```python
from build123d import *

# Parameters (mm, degrees)
SKETCH8_W                    = 28.7
SKETCH8_H                    = 15
BASE_FLANGE1_DEPTH           = 3.175
EDGE_FLANGE1_STRIP_W         = 16.7
EDGE_FLANGE1_STRIP_H         = 3.175
EDGE_FLANGE1_STRIP_CUT_DEPTH = 15
EDGE_FLANGE1_DEPTH           = 15
EDGE_FLANGE2_STRIP_W         = 16.7
EDGE_FLANGE2_STRIP_H         = 3.175
EDGE_FLANGE2_STRIP_CUT_DEPTH = 15
EDGE_FLANGE2_DEPTH           = 15
SKETCH19_R                   = 1.5
CUT_EXTRUDE1_DEPTH           = 10
CUT_EXTRUDE2_DEPTH           = 64.825465137
CUT_EXTRUDE2_DEPTH_BACK      = 64.825465137
CUT_EXTRUDE3_DEPTH           = 64.825465137
CUT_EXTRUDE3_DEPTH_BACK      = 64.825465137
SKETCH21_R                   = 1.5
FILLET1_R                    = 3


# Sheet-metal steps are written as plain solids
with BuildPart() as part:
    # Sketch8 → Base-Flange1 (new body)
    with BuildSketch(Plane(origin=(0, 0, 0), x_dir=(1, 0, 0), z_dir=(0, 1, 0))):
        with Locations((0, 7.5)):
            Rectangle(SKETCH8_W, SKETCH8_H)
    extrude(amount=-BASE_FLANGE1_DEPTH)

    # Edge-Flange1 strip (across the edge) → Edge-Flange1 strip cut (cut)
    with BuildSketch(Plane(origin=(14.35, -3.175, -15), x_dir=(-1, 0, 0), z_dir=(0, 0, 1))):
        with Locations((-3.175, -1.5875)):
            Rectangle(EDGE_FLANGE1_STRIP_W, EDGE_FLANGE1_STRIP_H)
    extrude(amount=EDGE_FLANGE1_STRIP_CUT_DEPTH, mode=Mode.SUBTRACT)

    # Edge-Flange1 section (across the edge) → Edge-Flange1 (add)
    with BuildSketch(Plane(origin=(14.35, -3.175, -15), x_dir=(-1, 0, 0), z_dir=(0, 0, 1))):
        with BuildLine():
            Line((0, 2), (0, 51.825))
            Line((0, 51.825), (3.175, 51.825))
            Line((3.175, 51.825), (3.175, 2))
            ThreePointArc((3.175, 2), (3.760786438, 0.585786438), (5.175, 0))
            Line((5.175, 0), (5.175, -3.175))
            ThreePointArc((5.175, -3.175), (1.515722407, -1.659277593), (0, 2))
        make_face()
    extrude(amount=EDGE_FLANGE1_DEPTH)

    # Edge-Flange2 strip (across the edge) → Edge-Flange2 strip cut (cut)
    with BuildSketch(Plane(origin=(-14.35, -3.175, 0), x_dir=(1, 0, 0), z_dir=(0, 0, -1))):
        with Locations((-3.175, -1.5875)):
            Rectangle(EDGE_FLANGE2_STRIP_W, EDGE_FLANGE2_STRIP_H)
    extrude(amount=EDGE_FLANGE2_STRIP_CUT_DEPTH, mode=Mode.SUBTRACT)

    # Edge-Flange2 section (across the edge) → Edge-Flange2 (add)
    with BuildSketch(Plane(origin=(-14.35, -3.175, 0), x_dir=(1, 0, 0), z_dir=(0, 0, -1))):
        with BuildLine():
            Line((0, 2), (0, 51.825))
            Line((0, 51.825), (3.175, 51.825))
            Line((3.175, 51.825), (3.175, 2))
            ThreePointArc((3.175, 2), (3.760786438, 0.585786438), (5.175, 0))
            Line((5.175, 0), (5.175, -3.175))
            ThreePointArc((5.175, -3.175), (1.515722407, -1.659277593), (0, 2))
        make_face()
    extrude(amount=EDGE_FLANGE2_DEPTH)

    # Sketch19 → Cut-Extrude1 (cut)
    with BuildSketch(Plane(origin=(0, 0, 0), x_dir=(1, 0, 0), z_dir=(0, 1, 0))):
        with Locations(Location((0, 7.5, 0), (0, 0, 270))):
            Circle(SKETCH19_R)
    extrude(amount=-CUT_EXTRUDE1_DEPTH, mode=Mode.SUBTRACT)

    # Sketch20 → Cut-Extrude2 (cut, two sides: drawn at the far end of the back side and taken through both)
    with BuildSketch(Plane(origin=(14.35, 0, 0), x_dir=(0, 0, -1), z_dir=(1, 0, 0)).offset(-CUT_EXTRUDE2_DEPTH_BACK)):
        Polygon((11.5, -55), (15, -5.175), (15, -55), align=None)
        Polygon((3.5, -55), (0, -5.175), (0, -55), align=None)
    extrude(amount=CUT_EXTRUDE2_DEPTH + CUT_EXTRUDE2_DEPTH_BACK, mode=Mode.SUBTRACT)

    # Sketch21 → Cut-Extrude3 (cut, two sides: drawn at the far end of the back side and taken through both)
    with BuildSketch(Plane(origin=(14.35, 0, 0), x_dir=(0, 0, -1), z_dir=(1, 0, 0)).offset(-CUT_EXTRUDE3_DEPTH_BACK)):
        with Locations(Location((7.5, -50.5, 0), (0, 0, 90))):
            Circle(SKETCH21_R)
    extrude(amount=CUT_EXTRUDE3_DEPTH + CUT_EXTRUDE3_DEPTH_BACK, mode=Mode.SUBTRACT)

    # Fillet1
    fillet1_edges = [part.edges().sort_by_distance(p)[0] for p in [
        (12.7625, -55, -3.5),
        (12.7625, -55, -11.5),
        (-12.7625, -55, -3.5),
        (-12.7625, -55, -11.5),
    ]]
    fillet(fillet1_edges, radius=FILLET1_R)


solid = part.part
```
The listing builds one solid part. Answer for the finished solid, in the listing's coordinates (mm). A direction names the side the tool comes from. Coordinates: 2 decimals unless noted, no trailing zeros. Write each loop counter-clockwise with the first axis right and the second up, starting at its lowest first coordinate (ties: lowest second). Pieces come first, ordered by that corner, then holes. Notation, with made-up numbers: (53.5, 89) -> (82.5, 89) arc R6 ccw to (82.5, 96) -> close; hole circle Ø6 at (19.5, -21). An arc over 180 degrees is marked (long way). Write each question's results on one line, items separated by ' | '. Start each with the question number.
1) A flat-ended cylindrical pin translates along its axis: pin 1 Ø4 at (x, z) = (0, -7.5) entering from -Y (3 decimals). Find the tip coordinate at first contact, or state that the pin passes through.
2) A cutting plane is placed at A-A (z = -7.5). Determine the outline of the cut face in (x, y) (3 decimals).
3) A tool of negligible diameter and unlimited length cuts with its end or side. For faces 1 (the flat face through (-11.175, -30, -7)), 2 (the cylindrical face through (-12.74, -54.173, -4.228)), from which of +Z, -Z, +X, -X, +Y, -Y can it reach the whole face along a straight path? Write none if from no direction.
4) For a pull along X with two mould halves and no side action, classify faces 3 (the cylindrical face through (12.794, -1.476, -7.605)), 4 (the flat face through (11.175, -30, -8)), 5 (the cylindrical face through (12.7, -51.7, -8.4)) as +X half, -X half, draft (parallel to the pull), parting line (faces both ways), or undercut.
5) A cutting plane is placed at D-D (x = 7.5). Determine the outline of the cut face in (y, z) (3 decimals), then the cut area to 3 significant figures.
6) Straight lines are drawn through the part: probe 1 along X at (y, z) = (-32, -4) (3 decimals); probe 2 along Y at (x, z) = (-4.25, -4.5) (3 decimals); probe 3 along X at (y, z) = (-1.35, -7.5). For each, find the intervals that lie inside material, in ascending order.
7) A cutting plane is placed at B-B (x = 0). Determine the outline of the cut face in (y, z) (3 decimals), then the cut area to 3 significant figures.
8) A cutting plane is placed at C-C (y = -46.5). Determine the outline of the cut face in (x, z) (3 decimals), then the cut area to 3 significant figures.
Values follow:
1) pin 1: y = -3.175
2) outline: (-14.35, -55) -> (-11.175, -55) -> (-11.175, -52) -> (-14.35, -52) -> close; (-14.35, -49) -> (-11.175, -49) -> (-11.175, -5.175) arc R2 cw to (-9.175, -3.175) -> (-1.5, -3.175) -> (-1.5, 0) -> (-9.175, 0) arc R5.175 ccw to (-14.35, -5.175) -> close; (1.5, -3.175) -> (9.175, -3.175) arc R2 cw to (11.175, -5.175) -> (11.175, -49) -> (14.35, -49) -> (14.35, -5.175) arc R5.175 ccw to (9.175, 0) -> (1.5, 0) -> close; (11.175, -55) -> (14.35, -55) -> (14.35, -52) -> (11.175, -52) -> close
3) face 1: +Z, -Z, -Y | face 2: +Z, +X, -X, -Y
4) face 3: +X half | face 4: undercut | face 5: draft
5) outline: (-3.175, -15) -> (0, -15) -> (0, 0) -> (-3.175, 0) -> close | area: 47.6 mm²
6) probe 1: -14.35 to -11.175, 11.175 to 14.35 | probe 2: -3.175 to 0 | probe 3: -12.66 to -1.5, 1.5 to 12.66
7) outline: (-3.175, -15) -> (0, -15) -> (0, -9) -> (-3.175, -9) -> close; (-3.175, -6) -> (0, -6) -> (0, 0) -> (-3.175, 0) -> close | area: 38.1 mm²
8) outline: (-14.35, -12.097) -> (-11.175, -12.097) -> (-11.175, -2.903) -> (-14.35, -2.903) -> close; (11.175, -12.097) -> (14.35, -12.097) -> (14.35, -2.903) -> (11.175, -2.903) -> close | area: 58.4 mm²
